from build123d import *

# Parameters (mm, degrees)
SKETCH1_W               = 13
SKETCH1_H               = 60
SKETCH1_R               = 2.05
BOSS_EXTRUDE1_DEPTH     = 2
SKETCH2_W               = 4
SKETCH2_H               = 60
BOSS_EXTRUDE2_DEPTH     = 15
SKETCH3_W               = 46
SKETCH3_H               = 90.1
BOSS_EXTRUDE3_DEPTH     = 3
MIRROR1_START           = 17
MIRROR1_DEPTH           = 3
MIRROR1_2_OUTLINE_W     = 4
MIRROR1_2_OUTLINE_H     = 60
MIRROR1_2_DEPTH         = 17
MIRROR1_3_OUTLINE_W     = 9
MIRROR1_3_OUTLINE_H     = 60
MIRROR1_3_OUTLINE_R     = 2.05
MIRROR1_3_DEPTH         = 2
SKETCH4_W               = 80
SKETCH4_H               = 5
CUT_EXTRUDE1_DEPTH      = 3
LPATTERN1_COUNT         = 8
LPATTERN1_PITCH         = 10
MIRROR2_COPY_1_SKETCH_W = 80
MIRROR2_COPY_1_SKETCH_H = 5
MIRROR2_COPY_1_DEPTH    = 3
MIRROR2_COPY_2_SKETCH_W = 80
MIRROR2_COPY_2_SKETCH_H = 5
MIRROR2_COPY_2_DEPTH    = 3
MIRROR2_COPY_3_SKETCH_W = 80
MIRROR2_COPY_3_SKETCH_H = 5
MIRROR2_COPY_3_DEPTH    = 3
MIRROR2_COPY_4_SKETCH_W = 80
MIRROR2_COPY_4_SKETCH_H = 5
MIRROR2_COPY_4_DEPTH    = 3
MIRROR2_COPY_5_SKETCH_W = 80
MIRROR2_COPY_5_SKETCH_H = 5
MIRROR2_COPY_5_DEPTH    = 3
MIRROR2_COPY_6_SKETCH_W = 80
MIRROR2_COPY_6_SKETCH_H = 5
MIRROR2_COPY_6_DEPTH    = 3
MIRROR2_COPY_7_SKETCH_W = 80
MIRROR2_COPY_7_SKETCH_H = 5
MIRROR2_COPY_7_DEPTH    = 3
FILLET1_R               = 1
SKETCH5_W               = 25
SKETCH5_H               = 5
BOSS_EXTRUDE4_DEPTH     = 17


# Read off the part's stored shape, not the designer's step: Mirror1
with BuildPart() as part:
    # Sketch1 → Boss-Extrude1 (new body)
    with BuildSketch(Plane(origin=(0, 0, 0), x_dir=(1, 0, 0), z_dir=(0, 1, 0))):
        with Locations((48.5, 60.1)):
            Rectangle(SKETCH1_W, SKETCH1_H)
        with Locations(Location((50, 77.1, 0), (0, 0, 270))):
            Circle(SKETCH1_R, mode=Mode.SUBTRACT)
        with Locations(Location((50, 60.1, 0), (0, 0, 270))):
            Circle(SKETCH1_R, mode=Mode.SUBTRACT)
        with Locations(Location((50, 35, 0), (0, 0, 270))):
            Circle(SKETCH1_R, mode=Mode.SUBTRACT)
    extrude(amount=BOSS_EXTRUDE1_DEPTH)

    # Sketch2 → Boss-Extrude2 (add)
    with BuildSketch(Plane(origin=(0, 2, 0), x_dir=(1, 0, 0), z_dir=(0, 1, 0))):
        with Locations((44, 60.1)):
            Rectangle(SKETCH2_W, SKETCH2_H)
    extrude(amount=BOSS_EXTRUDE2_DEPTH)

    # Sketch3 → Boss-Extrude3 (add)
    with BuildSketch(Plane(origin=(0, 17, 0), x_dir=(1, 0, 0), z_dir=(0, 1, 0))):
        with Locations((23, 45.05)):
            Rectangle(SKETCH3_W, SKETCH3_H)
    extrude(amount=BOSS_EXTRUDE3_DEPTH)

    # Mirror1 outline → Mirror1 (add)
    with BuildSketch(Plane(origin=(0, 0, 0), x_dir=(1, 0, 0), z_dir=(0, 1, 0)).offset(MIRROR1_START)):
        Polygon((46, -90.1), (46, 0), (0, 0), (0, 90.1), (-46, 90.1), (-46, -90.1), align=None)
    extrude(amount=MIRROR1_DEPTH)

    # Mirror1 2 outline → Mirror1 2 (add)
    with BuildSketch(Plane(origin=(0, 0, 0), x_dir=(1, 0, 0), z_dir=(0, 1, 0))):
        with Locations((44, -60.1)):
            Rectangle(MIRROR1_2_OUTLINE_W, MIRROR1_2_OUTLINE_H)
        with Locations((-44, -60.1)):
            Rectangle(MIRROR1_2_OUTLINE_W, MIRROR1_2_OUTLINE_H)
        with Locations((-44, 60.1)):
            Rectangle(MIRROR1_2_OUTLINE_W, MIRROR1_2_OUTLINE_H)
    extrude(amount=MIRROR1_2_DEPTH)

    # Mirror1 3 outline → Mirror1 3 (add)
    # profile 1 of 3: a face of its own
    with BuildSketch(Plane(origin=(0, 0, 0), x_dir=(1, 0, 0), z_dir=(0, 1, 0))):
        with Locations((50.5, -60.1)):
            Rectangle(MIRROR1_3_OUTLINE_W, MIRROR1_3_OUTLINE_H)
        with Locations((50, -77.1)):
            Circle(MIRROR1_3_OUTLINE_R, mode=Mode.SUBTRACT)
        with Locations((50, -60.1)):
            Circle(MIRROR1_3_OUTLINE_R, mode=Mode.SUBTRACT)
        with Locations((50, -35)):
            Circle(MIRROR1_3_OUTLINE_R, mode=Mode.SUBTRACT)
    # profile 2 of 3: a face of its own
    with BuildSketch(Plane(origin=(0, 0, 0), x_dir=(1, 0, 0), z_dir=(0, 1, 0))):
        with Locations((-50.5, -60.1)):
            Rectangle(MIRROR1_3_OUTLINE_W, MIRROR1_3_OUTLINE_H)
        with Locations((-50, -77.1)):
            Circle(MIRROR1_3_OUTLINE_R, mode=Mode.SUBTRACT)
        with Locations((-50, -60.1)):
            Circle(MIRROR1_3_OUTLINE_R, mode=Mode.SUBTRACT)
        with Locations((-50, -35)):
            Circle(MIRROR1_3_OUTLINE_R, mode=Mode.SUBTRACT)
    # profile 3 of 3: a face of its own
    with BuildSketch(Plane(origin=(0, 0, 0), x_dir=(1, 0, 0), z_dir=(0, 1, 0))):
        with Locations((-50.5, 60.1)):
            Rectangle(MIRROR1_3_OUTLINE_W, MIRROR1_3_OUTLINE_H)
        with Locations((-50, 35)):
            Circle(MIRROR1_3_OUTLINE_R, mode=Mode.SUBTRACT)
        with Locations((-50, 60.1)):
            Circle(MIRROR1_3_OUTLINE_R, mode=Mode.SUBTRACT)
        with Locations((-50, 77.1)):
            Circle(MIRROR1_3_OUTLINE_R, mode=Mode.SUBTRACT)
    extrude(amount=MIRROR1_3_DEPTH)

    # Sketch4 → Cut-Extrude1 (cut)
    with BuildSketch(Plane(origin=(0, 20, 0), x_dir=(1, 0, 0), z_dir=(0, 1, 0))):
        with Locations((0, 77.6)):
            Rectangle(SKETCH4_W, SKETCH4_H)
    cut_extrude1 = extrude(amount=-CUT_EXTRUDE1_DEPTH, mode=Mode.SUBTRACT)

    # LPattern1: Cut-Extrude1 ×8
    with Locations(*[(0, 0, i * LPATTERN1_PITCH) for i in range(1, LPATTERN1_COUNT)]):
        add(cut_extrude1, mode=Mode.SUBTRACT)

    # Mirror2: Cut-Extrude1 across Front Plane
    add(cut_extrude1.mirror(Plane.XY), mode=Mode.SUBTRACT)

    # Mirror2 copy 1 sketch → Mirror2 copy 1 (cut)
    with BuildSketch(Plane(origin=(0, 20, -10), x_dir=(1, 0, 0), z_dir=(0, 1, 0))):
        with Locations((0, -77.6)):
            Rectangle(MIRROR2_COPY_1_SKETCH_W, MIRROR2_COPY_1_SKETCH_H)
    extrude(amount=-MIRROR2_COPY_1_DEPTH, mode=Mode.SUBTRACT)

    # Mirror2 copy 2 sketch → Mirror2 copy 2 (cut)
    with BuildSketch(Plane(origin=(0, 20, -20), x_dir=(1, 0, 0), z_dir=(0, 1, 0))):
        with Locations((0, -77.6)):
            Rectangle(MIRROR2_COPY_2_SKETCH_W, MIRROR2_COPY_2_SKETCH_H)
    extrude(amount=-MIRROR2_COPY_2_DEPTH, mode=Mode.SUBTRACT)

    # Mirror2 copy 3 sketch → Mirror2 copy 3 (cut)
    with BuildSketch(Plane(origin=(0, 20, -30), x_dir=(1, 0, 0), z_dir=(0, 1, 0))):
        with Locations((0, -77.6)):
            Rectangle(MIRROR2_COPY_3_SKETCH_W, MIRROR2_COPY_3_SKETCH_H)
    extrude(amount=-MIRROR2_COPY_3_DEPTH, mode=Mode.SUBTRACT)

    # Mirror2 copy 4 sketch → Mirror2 copy 4 (cut)
    with BuildSketch(Plane(origin=(0, 20, -40), x_dir=(1, 0, 0), z_dir=(0, 1, 0))):
        with Locations((0, -77.6)):
            Rectangle(MIRROR2_COPY_4_SKETCH_W, MIRROR2_COPY_4_SKETCH_H)
    extrude(amount=-MIRROR2_COPY_4_DEPTH, mode=Mode.SUBTRACT)

    # Mirror2 copy 5 sketch → Mirror2 copy 5 (cut)
    with BuildSketch(Plane(origin=(0, 20, -50), x_dir=(1, 0, 0), z_dir=(0, 1, 0))):
        with Locations((0, -77.6)):
            Rectangle(MIRROR2_COPY_5_SKETCH_W, MIRROR2_COPY_5_SKETCH_H)
    extrude(amount=-MIRROR2_COPY_5_DEPTH, mode=Mode.SUBTRACT)

    # Mirror2 copy 6 sketch → Mirror2 copy 6 (cut)
    with BuildSketch(Plane(origin=(0, 20, -60), x_dir=(1, 0, 0), z_dir=(0, 1, 0))):
        with Locations((0, -77.6)):
            Rectangle(MIRROR2_COPY_6_SKETCH_W, MIRROR2_COPY_6_SKETCH_H)
    extrude(amount=-MIRROR2_COPY_6_DEPTH, mode=Mode.SUBTRACT)

    # Mirror2 copy 7 sketch → Mirror2 copy 7 (cut)
    with BuildSketch(Plane(origin=(0, 20, -70), x_dir=(1, 0, 0), z_dir=(0, 1, 0))):
        with Locations((0, -77.6)):
            Rectangle(MIRROR2_COPY_7_SKETCH_W, MIRROR2_COPY_7_SKETCH_H)
    extrude(amount=-MIRROR2_COPY_7_DEPTH, mode=Mode.SUBTRACT)

    # Fillet1
    fillet1_edges = [part.edges().sort_by_distance(p)[0] for p in [
        (46, 2, -60.1),
        (46, 20, 0),
        (0, 20, -90.1),
        (-46, 2, -60.1),
        (-46, 2, 60.1),
        (-46, 20, 0),
        (46, 2, 60.1),
        (0, 20, 90.1),
    ]]
    fillet(fillet1_edges, radius=FILLET1_R)

    # Sketch5 → Boss-Extrude4 (add)
    with BuildSketch(Plane.XZ.offset(-17)):
        with Locations((0, 22.6)):
            Rectangle(SKETCH5_W, SKETCH5_H)
        with Locations((0, -22.6)):
            Rectangle(SKETCH5_W, SKETCH5_H)
    extrude(amount=BOSS_EXTRUDE4_DEPTH)


solid = part.part
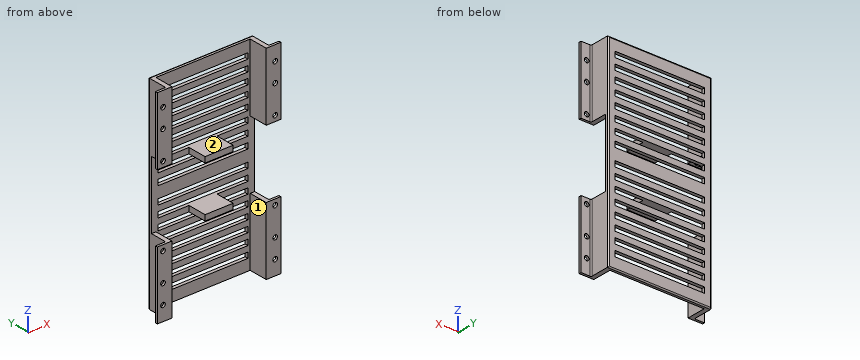
Can you work these out from the model? Positions are in its coordinate system, mm. Face numbers are marked on the shaded views. A direction names the side the tool comes from. Give positions to 0.01 mm unless a question says otherwise; leave off trailing zeros. Loops run counter-clockwise (first coordinate to the right, second up) from the corner with the lowest first, then second, coordinate; pieces in that order, holes last. Notation, with made-up numbers: (12.25, 71) -> (39.25, 71) arc R25 cw to (39.25, 99) -> close; hole circle Ø1 at (86.25, 0). An arc over 180 degrees is marked (long way). Use one line per item in the form item = value.
1) Will these pins go through, and if not, where does the flat tip stop? pin 1 (0.9 mm diameter, centred on y = 18.5, z = -7, fed in from -X); pin 2 (1.5 mm diameter, centred on x = 4.5, y = 15.5, fed in from -Z); pin 3 (2.5 mm diameter, centred on y = 19, z = -8, fed in from +X).
Answers:
pin_1 = -46
pin_2 = -25.1
pin_3 = 46
2) If we section it at B-B (x = -50): Count the separate pieces of the cut face and the enclosed holes in it, plus the area to 3 significant figures.
Answers:
separate_pieces = 8
enclosed_holes = 0
area = 191 mm²
3) If we section it at A-A (z = -77.1): Please give me the cut outline in (x, y), plus the area to 3 significant figures.
Answers:
outline = (-55, 0) -> (-52.05, 0) -> (-52.05, 2) -> (-55, 2) -> close; (-47.95, 0) -> (-42, 0) -> (-42, 17) -> (-40, 17) -> (-40, 20) -> (-45, 20) arc R1 ccw to (-46, 19) -> (-46, 3) arc R1 cw to (-47, 2) -> (-47.95, 2) -> close; (40, 17) -> (42, 17) -> (42, 0) -> (47.95, 0) -> (47.95, 2) -> (47, 2) arc R1 cw to (46, 3) -> (46, 19) arc R1 ccw to (45, 20) -> (40, 20) -> close; (52.05, 0) -> (55, 0) -> (55, 2) -> (52.05, 2) -> close
area = 192 mm²
4) If we section it at D-D (z = 52): Please give me the cut outline in (x, y).
Answers:
outline = (-55, 0) -> (-42, 0) -> (-42, 17) -> (42, 17) -> (42, 0) -> (55, 0) -> (55, 2) -> (47, 2) arc R1 cw to (46, 3) -> (46, 19) arc R1 ccw to (45, 20) -> (-45, 20) arc R1 ccw to (-46, 19) -> (-46, 3) arc R1 cw to (-47, 2) -> (-55, 2) -> close
5) For the marked faces 1 and 2, which set-ups out of +Z, -Z, +X, -X, +Y, -Y let a thin tool reach every point of the face, with its end or its side?
Answers:
face_1 = +Z, -Z, -Y
face_2 = +Y, -Y
6) I need wall thicknesses on line 1 along X through (y, z) = (1.35, -77.1); line 2 along Z through (x, y) = (-3, 12.25); line 3 along X through (y, z) = (18.75, -68.5). Which ranges of each line are inside material? Lowest first, please.
Answers:
line_1 = -55 to -52.05, -47.95 to -42, 42 to 47.95, 52.05 to 55
line_2 = -25.1 to -20.1, 20.1 to 25.1
line_3 = -46 to -40, 40 to 46
7) If we section it at C-C (y = 13.5): Please give me the cut outline in (x, z).
Answers:
outline = (-46, -90.1) -> (-42, -90.1) -> (-42, -30.1) -> (-46, -30.1) -> close; (-46, 30.1) -> (-42, 30.1) -> (-42, 90.1) -> (-46, 90.1) -> close; (-12.5, -25.1) -> (12.5, -25.1) -> (12.5, -20.1) -> (-12.5, -20.1) -> close; (-12.5, 20.1) -> (12.5, 20.1) -> (12.5, 25.1) -> (-12.5, 25.1) -> close; (42, -90.1) -> (46, -90.1) -> (46, -30.1) -> (42, -30.1) -> close; (42, 30.1) -> (46, 30.1) -> (46, 90.1) -> (42, 90.1) -> close
